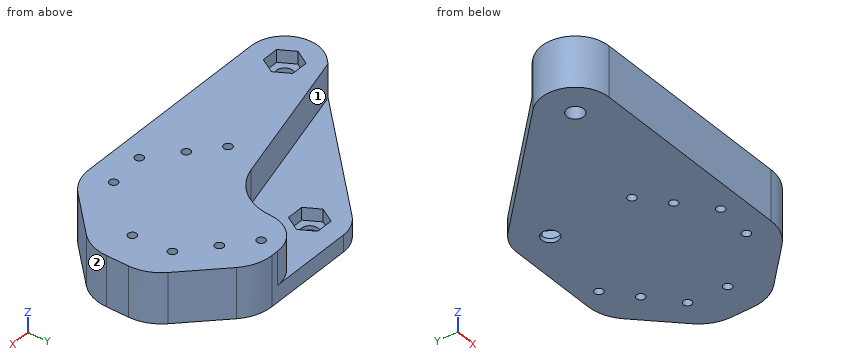
Autodesk Inventor part; units mm, degrees
ref_plane "YZ Plane" through (0, 0, 0) normal (1, 0, 0) x (0, 1, 0)
ref_plane "XZ Plane" through (0, 0, 0) normal (0, 1, 0) x (-1, 0, 0)
ref_plane "XY Plane" through (0, 0, 0) normal (0, 0, 1) x (1, 0, 0)
sketch "Esquisse1" plane through (0, 0, 0) normal (0, 0, 1) x (1, 0, 0)
  line L0 (0, 0) -> (52, 0) construction
  line L1 (0, 0) -> (27.5772, 27.5772) construction
  circle A0 centre (27.5772, 27.5772) radius 2
  circle A1 centre (0, 0) radius 2
  line L2 (0, 0) -> (0, -8) construction
  line L3 (0, 0) -> (-5.6569, 5.6569) construction
  line L4 (68.4653, -8) -> (-19.3137, -8)
  line L5 (27.5772, 27.5772) -> (27.5772, 35.5772) construction
  line L6 (-19.3137, -8) -> (24.2635, 35.5772)
  line L7 (24.2635, 35.5772) -> (68.4653, 35.5772)
  line L8 (27.5772, 27.5772) -> (49, 27.5772) construction
  line L9 (27.5772, 27.5772) -> (55.0016, 4.5654) construction
  line L10 (27.5772, 27.5772) -> (37.219, 39.0678) construction
  line L11 (37.219, 39.0678) -> (41.8152, 35.2111) construction
  line L12 (41.8152, 35.2111) -> (46.7945, 31.033) construction
  line L13 (46.7945, 31.033) -> (52.9229, 25.8907) construction
  line L14 (52.9229, 25.8907) -> (59.8173, 20.1056) construction
  line L15 (55.0016, 4.5654) -> (60.4653, 11.0767) construction
  circle A2 centre (41.8152, 35.2111) radius 1 construction
  circle A3 centre (46.7945, 31.033) radius 1
  circle A4 centre (52.9229, 25.8907) radius 1
  circle A5 centre (59.8173, 20.1056) radius 1
  circle A6 centre (60.4653, 11.0767) radius 1
  circle A7 centre (22.5316, 12.2298) radius 1 construction
  circle A8 centre (27.5109, 8.0517) radius 1
  circle A9 centre (33.6393, 2.9094) radius 1
  circle A10 centre (40.5337, -2.8757) radius 1
  circle A11 centre (49.5379, -1.946) radius 1
  line L16 (60.4653, 11.0767) -> (68.4653, 11.0767) construction
  line L17 (68.4653, 35.5772) -> (68.4653, -8)
  dimension "d39" = 39
  dimension "d41" = 4
  dimension "d44" = 8
  dimension "d64" = 8
  dimension "d80" = 45
  dimension "d82" = 8
  dimension "d101" = 35.8
  dimension "d102" = 40
  dimension "d103" = 15
  dimension "d104" = 6
  dimension "d105" = 6.5
  dimension "d106" = 8
  dimension "d107" = 9
  dimension "d108" = 8.5
  dimension "d109" = 2
  dimension "d110" = 8
extrude "Extrusion15" add sketch "Esquisse1" along normal blind 12
sketch "Esquisse13" plane through (0, 0, 12) normal (0, 0, 1) x (1, 0, 0)
  circle A0 centre (0, 0) radius 2
  circle A1 centre (27.5772, 27.5772) radius 2
  line L0 (68.4653, -8) -> (68.4653, 35.5772)
  line L1 (68.4653, 35.5772) -> (24.2635, 35.5772)
  line L2 (24.2635, 35.5772) -> (-19.3137, -8)
  circle A2 centre (27.5772, 27.5772) radius 12 construction
  line L3 (39.5772, 35.5772) -> (39.5772, 27.5772)
  line L4 (0, 0) -> (0, 8) construction
  line L5 (-4.4796, 6.8341) -> (30.5997, 15.964)
  arc A3 (30.5997, 15.964) -> (39.5772, 27.5772) centre (27.5772, 27.5772) ccw
  dimension "d128" = 24
  dimension "d129" = 8
extrude "Extrusion16" cut sketch "Esquisse13" against normal blind 8 contours L3 A3 L5 L2 L1
sketch "Esquisse14" plane through (0, 0, 12) normal (0, 0, 1) x (1, 0, 0)
  line L0 (-19.3137, -8) -> (68.4653, -8)
  circle A0 centre (0, 0) radius 2
  line L1 (4.0415, 0) -> (2.0207, -3.5)
  line L2 (2.0207, -3.5) -> (-2.0207, -3.5)
  line L3 (-2.0207, -3.5) -> (-4.0415, 0)
  line L4 (-4.0415, 0) -> (-2.0207, 3.5)
  line L5 (-2.0207, 3.5) -> (2.0207, 3.5)
  line L6 (2.0207, 3.5) -> (4.0415, 0)
  line L7 (2.0207, 3.5) -> (2.0207, -3.5) construction
  dimension "d132" = 7
sketch "Esquisse15" plane through (0, 0, 4) normal (0, 0, 1) x (1, 0, 0)
  circle A0 centre (27.5772, 27.5772) radius 2
  arc A1 (30.5997, 15.964) -> (39.5772, 27.5772) centre (27.5772, 27.5772) ccw
  line L0 (31.6186, 27.5772) -> (29.5979, 24.0772)
  line L1 (29.5979, 24.0772) -> (25.5564, 24.0772)
  line L2 (25.5564, 24.0772) -> (23.5357, 27.5772)
  line L3 (23.5357, 27.5772) -> (25.5564, 31.0772)
  line L4 (25.5564, 31.0772) -> (29.5979, 31.0772)
  line L5 (29.5979, 31.0772) -> (31.6186, 27.5772)
  line L6 (-19.3137, -8) -> (68.4653, -8)
  line L7 (-2.0207, 3.5) -> (2.0207, 3.5)
  point P0 (0, 0)
extrude "Extrusion17" cut sketch "Esquisse14" against normal blind 3
extrude "Extrusion18" cut sketch "Esquisse15" against normal blind 3
fillet "Congé8" radius 8 1 edges at (-19.3137, -8, 6)
fillet "Congé9" radius 8 1 edges at (24.2635, 35.5772, 2)
fillet "Congé10" radius 8 1 edges at (39.5772, 35.5772, 8)
chamfer "Chanfrein1" distance 15 angle 45 1 edges at (68.4653, 35.5772, 6)
chamfer "Chanfrein2" distance 15 angle 45 1 edges at (68.4653, -8, 6)
fillet "Congé12" radius 10 1 edges at (53.4653, -8, 6)
fillet "Congé13" radius 10 1 edges at (68.4653, 7, 6)
fillet "Congé14" radius 10 1 edges at (68.4653, 20.5772, 6)
fillet "Congé15" radius 10 1 edges at (53.4653, 35.5772, 6)
properties part number "joint1+mx28imprint_v2"
Design review of the part built by this model. Coordinates are the model's own, in mm. Face numbers are marked on the shaded views. A direction names the side the tool comes from. Coordinates: 2 decimals unless noted, no trailing zeros. Order: outer loops, then holes, each group sorted by start corner. A loop starts at its lowest first (then second) coordinate and runs counter-clockwise, first axis right, second up.
Item 1: Take a section at A-A, the plane z = 10.5. Count the separate pieces of the cut face and the enclosed holes in it, then the cut area to 3 significant figures.
Item 2: For pin 1 Ø4 at (x, z) = (37.5, 5.5) entering from +Y; pin 2 Ø0.9 at (x, z) = (-0.5, 10.5) entering from +Y; pin 3 Ø2 at (x, y) = (25.5, 28.5) entering from +Z; pin 4 Ø4 at (x, z) = (60, 10.5) entering from -Y, all flat-tipped, find the tip position at first contact; note any pin that passes through.
Item 3: For line 1 (Y direction, x = 60.5, z = 6.5); line 2 (Y direction, x = 50, z = 2); line 3 (Y direction, x = 0, z = 4.25), list the stretches that pass through material, from the lowest coordinate up.
Item 4: For the marked faces 1 and 2, list the 3-axis set-ups (+Z, -Z, +X, -X, +Y, -Y) from which the entire face can be reached by the end or side of a thin tool; tool diameter is ignored.
Item 5: Take a section at B-B, the plane x = 16. Write out the cut boundary in (y, z), then the cut area to 3 significant figures.
The answers:
1. separate pieces: 1
1. enclosed holes: 9
1. area: 1,900 mm2
2. pin 1: stops at y = 35.58
2. pin 2: stops at y = 7.99
2. pin 3: stops at z = 1
2. pin 4: stops at y = -3.47
3. line 1: y = -0.97 to 10.08, 12.08 to 19.37, 20.84 to 28.54
3. line 2: y = -7.98 to -2.83, -1.06 to 35.55
3. line 3: y = -8 to -2, 2 to 8
4. face 1: +Z, -X, +Y
4. face 2: +Z, -Z, +X, -Y
5. outline: (-8, 0) - (27.31, 0) - (27.31, 4) - (12.16, 4) - (12.16, 12) - (-8, 12) - close
5. area: 303 mm2
